Geometry: final body of the model. Coordinates: model frame, mm. A direction names the side the tool comes from. Give positions to 0.01 mm unless a question says otherwise; leave off trailing zeros. Order: outer loops, then holes, each group sorted by start corner. A loop starts at its lowest first (then second) coordinate and runs counter-clockwise, first axis right, second up. Notation, with made-up numbers: (76, -3) -> (110, -3) arc R21 ccw to (110, 1) -> close; hole circle Ø2 at (-27.75, 23). An arc over 180 degrees is marked (long way). One line per question, with ' | ' between items.
Autodesk Inventor part; units mm, degrees
ref_plane "YZ Plane" through (0, 0, 0) normal (1, 0, 0) x (0, 1, 0)
ref_plane "XZ Plane" through (0, 0, 0) normal (0, 1, 0) x (-1, 0, 0)
ref_plane "XY Plane" through (0, 0, 0) normal (0, 0, 1) x (1, 0, 0)
sketch "スケッチ1" plane through (0, 0, 0) normal (0, 0, 1) x (1, 0, 0)
  circle A0 centre (0, 0) radius 10.5 construction
  circle A1 centre (-13.5, 1) radius 1.35
  line L0 (-13.5, 28) -> (13.5, 28) construction
  line L1 (13.5, 28) -> (13.5, 1) construction
  line L2 (13.5, 1) -> (-13.5, 1) construction
  line L3 (-13.5, 1) -> (-13.5, 28) construction
  circle A2 centre (-13.5, 28) radius 1.35
  circle A3 centre (13.5, 1) radius 1.35
  circle A4 centre (13.5, 28) radius 1.35
  line L4 (-16.25, 10) -> (-16.25, 7.1)
  line L5 (-16.25, 10) -> (16.25, 10)
  line L6 (16.25, 10) -> (16.25, 7.1)
  line L7 (-16.25, -7.1) -> (-16.25, -10)
  line L8 (-16.25, -10) -> (16.25, -10)
  line L9 (16.25, -7.1) -> (16.25, -10)
  line L10 (-16.25, 5) -> (-17.75, 5)
  line L11 (-17.75, 5) -> (-17.75, -5)
  line L12 (-17.75, -5) -> (-16.25, -5)
  arc A5 (-16.25, 5) -> (-16.25, 7.1) centre (-16.25, 6.05) ccw
  arc A6 (-16.25, -7.1) -> (-16.25, -5) centre (-16.25, -6.05) ccw
  line L13 (16.25, 5) -> (17.75, 5)
  line L14 (17.75, 5) -> (17.75, -5)
  line L15 (17.75, -5) -> (16.25, -5)
  arc A7 (16.25, 7.1) -> (16.25, 5) centre (16.25, 6.05) ccw
  line L16 (0, 28) -> (0, 0) construction
  arc A8 (16.25, -5) -> (16.25, -7.1) centre (16.25, -6.05) ccw
  line L17 (-17.75, 0) -> (17.75, 0) construction
  circle A9 centre (0, 0) radius 6.05
  point P0 (0, 10)
  dimension "d8" = 21
  dimension "d10" = 27
  dimension "d12" = 1
  dimension "d13" = 2.7
  dimension "d38" = 27
  dimension "d44" = 27
  dimension "d47" = 1.05
  dimension "d48" = 32.5
  dimension "d49" = 1.5
  dimension "d50" = 10
  dimension "d51" = 5
  dimension "d52" = 12.1
  dimension "d64" = 1.5
extrude "押し出し1" add sketch "スケッチ1" along normal blind 2 contours L5 L6 A7 L13 L14 L15 A8 L9 L8 L7 A6 L12 L11 L10 A5 L4
sketch "スケッチ3" plane through (0, 0, 2) normal (0, 0, 1) x (1, 0, 0)
  circle A0 centre (0, 0) radius 6.05
  circle A1 centre (13.5, 1) radius 1.35
  circle A2 centre (-13.5, 1) radius 1.35
  line L0 (16.25, 10) -> (-16.25, 10)
  line L1 (-11.154, 3.5) -> (-7.2493, 3.5)
  line L2 (-11.154, -1.5) -> (-7.909, -1.5)
  line L3 (-13.5, 1) -> (13.5, 1) construction
  arc A3 (7.2493, 3.5) -> (-7.2493, 3.5) centre (0, 0) ccw
  line L4 (7.2493, 3.5) -> (11.154, 3.5)
  line L5 (-14.3875, 13.5275) -> (14.3875, 13.5275)
  line L6 (0, 0) -> (0, 10) construction
  arc A4 (-7.909, -1.5) -> (7.909, -1.5) centre (0, 0) ccw
  line L7 (7.909, -1.5) -> (11.154, -1.5)
  line L8 (14.3875, -14.6128) -> (-14.3875, -14.6128)
  line L9 (-16.25, -10) -> (16.25, -10)
  line L10 (-14.3875, -14.6128) -> (-11.154, -1.5)
  line L11 (-11.154, 3.5) -> (-14.3875, 13.5275)
  circle A5 centre (-13.5, 1) radius 3 construction
  line L12 (11.154, -1.5) -> (14.3875, -14.6128)
  line L13 (11.154, 3.5) -> (14.3875, 13.5275)
  line L14 (-13.25, 10) -> (-16.25, 10) construction
  line L15 (-13.25, -10) -> (-16.25, -10) construction
  line L16 (13.25, 10) -> (16.25, 10) construction
  line L17 (16.25, -10) -> (13.25, -10) construction
  dimension "d68" = 2.5
  dimension "d69" = 2
  dimension "d73" = 6
  dimension "d74" = 3
extrude "押し出し3" cut sketch "スケッチ3" against normal blind 10 contours L13 L4 A3 L1 L11 L0 | L2 A4 L7 L12 L9 L10
fillet "フィレット2" radius 2 12 edges at (-11.154, 3.5, 1) (-7.2493, 3.5, 1) (7.909, -1.5, 1) (7.2493, 3.5, 1) (11.154, 3.5, 1) (-7.909, -1.5, 1) (-11.154, -1.5, 1) (11.154, -1.5, 1) (-13.25, -10, 1) (-13.25, 10, 1) (13.25, -10, 1) (13.25, 10, 1)
equation "\"d38\" = d10"
equation "\"d44\" = d10"
equation "\"d50\" = d11"
equation "\"d51\" = d28"
equation "\"d64\" = d49"
equation "\"d11\" = 10"
equation "\"d28\" = 5"
properties part number "足首_サブフレーム_1_2" material "アルミニウム 2014-T4"
1) Section C-C on x = 13.5. Return loops of the section in (y, z), plus the area to 3 significant figures.
Check result:
outline: (-9.51, 0) -> (-0.35, 0) -> (-0.35, 2) -> (-9.51, 2) -> close; (2.35, 0) -> (9.6, 0) -> (9.6, 2) -> (2.35, 2) -> close | area: 32.8 mm^2
2) Set-up query: faces 1 (the flat face through (-15, 10, 1)), 2 (the cylindrical face through (-13.569, -9.563, 0.986)), 3 (the cylindrical face through (-10.9, 3.9, 1)), 4 (the flat face through (17, 5, 1)), 5 (the flat face through (17, -5, 1)). Return all of +Z, -Z, +X, -X, +Y, -Y with unobstructed straight access to the full face (end or side cutting, diameter ignored); none if empty.
Check result:
face 1: +Z, -Z, +X, -X, +Y | face 2: +Z, -Z, -Y | face 3: +Z, -Z, +Y | face 4: +Z, -Z, +X, +Y | face 5: +Z, -Z, +X, -Y
3) Contact query for flat-ended pins moving along their axis: pin 1 Ø1.2 at (x, z) = (-17, 1) entering from -Y; pin 2 Ø0.6 at (y, z) = (8.5, 1.5) entering from +X; pin 3 Ø1 at (x, z) = (9, 1) entering from +Y. Output: stop coordinate, or through.
Check result:
pin 1: stops at y = -5 | pin 2: stops at x = 16.25 | pin 3: stops at y = 3.5
4) Section D-D on z = 0.6. Count the separate pieces of the cut face and the enclosed holes in it, plus the area to 3 significant figures.
Check result:
separate pieces: 1 | enclosed holes: 3 | area: 307 mm^2
5) Material intervals for probe 1 along X at (y, z) = (-2, 0.95); probe 2 along X at (y, z) = (-3.5, 0.9); probe 3 along Y at (x, z) = (0, 1.5), sorted ascending. Write a range as from..to.
Check result:
probe 1: x = -17.75..-10.91, -8.1..-5.71, 5.71..8.1, 10.91..17.75 | probe 2: x = -17.75..-11.65, -7.25..-4.93, 4.93..7.25, 11.65..17.75 | probe 3: y = -8.05..-6.05, 6.05..8.05
6) Section B-B on y = 0. Return loops of the section in (x, z).
Check result:
outline: (-17.75, 0) -> (-14.41, 0) -> (-14.41, 2) -> (-17.75, 2) -> close; (-12.59, 0) -> (-6.05, 0) -> (-6.05, 2) -> (-12.59, 2) -> close; (6.05, 0) -> (12.59, 0) -> (12.59, 2) -> (6.05, 2) -> close; (14.41, 0) -> (17.75, 0) -> (17.75, 2) -> (14.41, 2) -> close
7) Pull-direction query (X, two-part tool) for faces 6 (the flat face through (16.25, -9, 1)), 7 (the flat face through (-17, 5, 1)), 8 (the flat face through (-12.21, -5.79, 1.01)); classes: +X half, -X half, draft (parallel to the pull), parting line (faces both ways), or undercut.
Check result:
face 6: +X half | face 7: draft | face 8: undercut
8) Section A-A on x = 0. Return loops of the section in (y, z).
Check result:
outline: (-8.05, 0) -> (-6.05, 0) -> (-6.05, 2) -> (-8.05, 2) -> close; (6.05, 0) -> (8.05, 0) -> (8.05, 2) -> (6.05, 2) -> close
